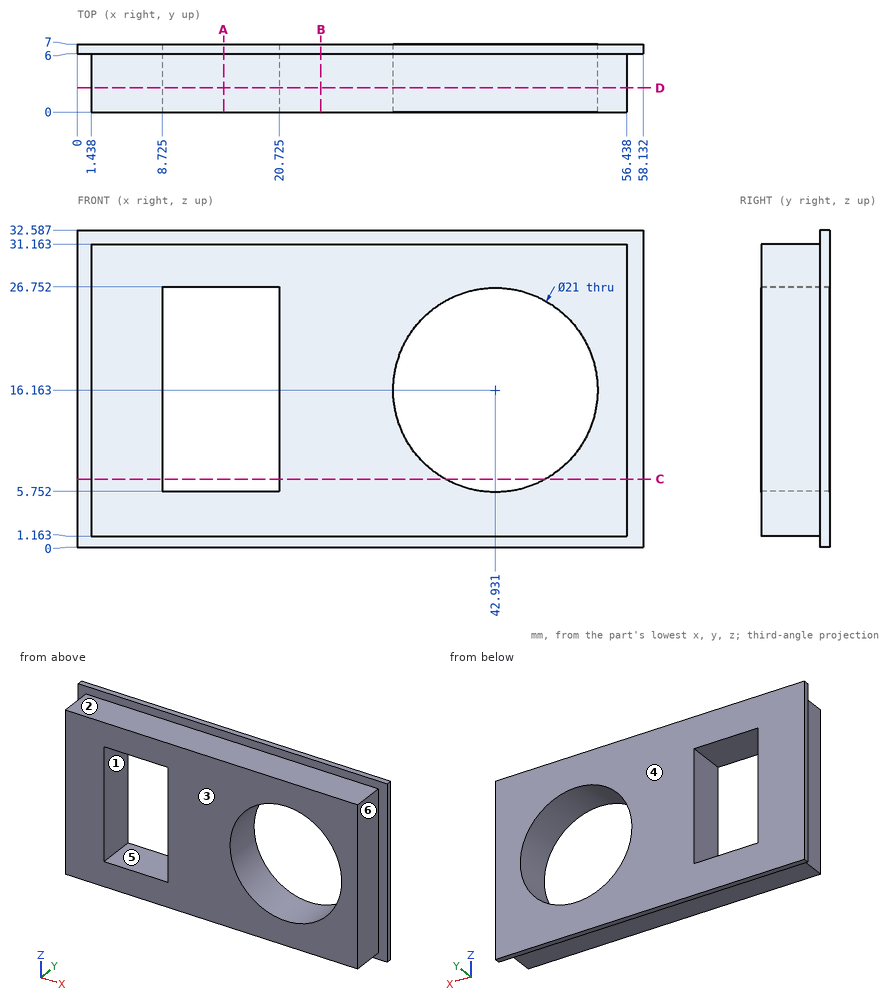
Study the drawing (mm; zero at the part's minimum x, y, z) and answer. A direction names the side the tool comes from. Give positions to 0.01 mm unless a question says otherwise; leave off trailing zeros. Write each loop counter-clockwise with the first axis right and the second up, starting at its lowest first coordinate (ties: lowest second). Pieces come first, ordered by that corner, then holes.
Item 1: Section D-D, the plane y = 2.5 is taken. Write down the section's boundary in (x, z) (1 decimal), plus the area to 3 significant figures.
Item 2: Flat-ended cylindrical pins translate along their axes: P1, Ø1, axis at x = 12, y = 3.5, coming from the +Z side; P2, Ø2, axis at y = 4.5, z = 11.5, coming from the +X side; P3, Ø1.8, axis at x = 18.5, y = 3.5, coming from the -Z side. Find the tip coordinate at first contact, or state that the pin passes through.
Item 3: Which of the six approach directions +Z, -Z, +X, -X, +Y, -Y give full straight-line access (tool end or side, diameter ignored) to the marked faces 4, 5 and 6?
Item 4: Determine the mould class of the marked faces 1, 2 and 3 for opening direction Z: released by +Z, released by -Z, zero draft, split by the parting line, or undercut.
Item 5: Section B-B, the plane x = 25 is taken. Write down the section's boundary in (y, z), plus the area to 3 significant figures.
Item 6: Find the intervals of material crossed by line 1 along X through (y, z) = (4, 12.5) (1 decimal); line 2 along X through (y, z) = (3.5, 10) (1 decimal); line 3 along Z through (x, y) = (17, 3), in increasing order.
Item 7: Section A-A, the plane x = 15 is taken. Write down the section's boundary in (y, z).
Item 8: Section C-C, the plane z = 7 is taken. Write down the section's boundary in (x, y) (1 decimal).
Completed:
1. outline: (1.4, 1.2) - (56.4, 1.2) - (56.4, 31.2) - (1.4, 31.2) - close; hole (8.7, 5.8) - (20.7, 5.8) - (20.7, 26.8) - (8.7, 26.8) - close; hole circle Ø21 at (42.9, 16.2)
1. area: 1,050 mm2
2. P1: stops at z = 31.16
2. P2: stops at x = 56.44
2. P3: stops at z = 1.16
3. face 4: +Z, -Z, +X, -X, +Y
3. face 5: +Y, -Y
3. face 6: +Z, -Z, +X, -Y
4. face 1: undercut
4. face 2: released by +Z
4. face 3: zero draft
5. outline: (0, 1.16) - (6, 1.16) - (6, 0) - (7, 0) - (7, 32.59) - (6, 32.59) - (6, 31.16) - (0, 31.16) - close
5. area: 213 mm2
6. line 1: x = 1.4 to 8.7, 20.7 to 33.1, 52.8 to 56.4
6. line 2: x = 1.4 to 8.7, 20.7 to 34.4, 51.4 to 56.4
6. line 3: z = 1.16 to 5.75, 26.75 to 31.16
7. outline: (0, 1.16) - (6, 1.16) - (6, 0) - (7, 0) - (7, 5.75) - (0, 5.75) - close; (0, 26.75) - (7, 26.75) - (7, 32.59) - (6, 32.59) - (6, 31.16) - (0, 31.16) - close
8. outline: (0, 6) - (1.4, 6) - (1.4, 0) - (8.7, 0) - (8.7, 7) - (0, 7) - close; (20.7, 0) - (37.8, 0) - (37.8, 7) - (20.7, 7) - close; (48.1, 0) - (56.4, 0) - (56.4, 6) - (58.1, 6) - (58.1, 7) - (48.1, 7) - close
